```python
from build123d import *

# Parameters (mm, degrees)
F1_DEPTH = 30
F2_R     = 6.223398
F2_R_2   = 5.996206
F2_R_3   = 6.721343
F2_R_4   = 6.043049
F3_DEPTH = 35
F4_R     = 17.538538
F5_DEPTH = 500


with BuildPart() as f1:
    # F0 (on Front) → F1 (new body)
    with BuildSketch(Plane.XZ):
        with BuildLine():
            Line((-400.257468, -150.029927), (400.257468, -150.029927))
            ThreePointArc((400.257468, -150.029927), (550.287396, 0), (400.257468, 150.029927))
            Line((400.257468, 150.029927), (-400.257468, 150.029927))
            Line((-400.257468, 150.029927), (-400.257468, -150.029927))
        make_face()
    extrude(amount=F1_DEPTH)

    # F2 (on face) → F3 (cut)
    with BuildSketch(Plane.XZ.offset(30)):
        with Locations((-361.057468, 135.091782)):
            Circle(F2_R)
        with Locations((-361.057468, 104.35146)):
            Circle(F2_R_2)
        with Locations((-137.267468, 135.091782)):
            Circle(F2_R_3)
        with Locations((-137.267468, 104.35146)):
            Circle(F2_R_4)
    extrude(amount=-F3_DEPTH, mode=Mode.SUBTRACT)

    # F4 (on Top) → F5 (cut, symmetric)
    with BuildSketch(Plane.XY):
        with Locations((-400.190324, -14.999421)):
            Circle(F4_R)
    extrude(amount=F5_DEPTH, both=True, mode=Mode.SUBTRACT)


solid = f1.part
```
Design review of the part built by this model. Coordinates are the model's own, in mm. Coordinates: 2 decimals unless noted, no trailing zeros. Write each loop counter-clockwise with the first axis right and the second up, starting at its lowest first coordinate (ties: lowest second). Pieces come first, ordered by that corner, then holes. Notation, with made-up numbers: M 14,65 L 18,65 A29 cw 18,95 Z; hole C 71.25,39 d9. An arc over 180 degrees is marked long. Answer as a JSON object with one key per item and string values.
Item 1: Draft analysis for pull direction Y (two halves, no side actions). For faces 1 (the flat face through (-1, -15, -150.03)), 2 (the cylindrical face through (-382.654, -15.252, 2.1)), 3 (the flat face through (73, -30, 2)), state which applies: pulls with the +Y half, pulls with the -Y half, needs draft (parallel to the pull), parting line crosses it, or undercut.
Outcome:
{"face 1": "needs draft", "face 2": "undercut", "face 3": "pulls with the -Y half"}
Item 2: Insertion check: pin 1 Ø8 at (y, z) = (-9, -95.5) entering from -X; pin 2 Ø8 at (x, z) = (-137.27, 135.09) entering from -Y; pin 3 Ø8 at (y, z) = (-20, -6) entering from -X. Each pin has a flat end and moves straight along its axis. Give the tip position at first contact, or say it passes through.
Outcome:
{"pin 1": "x = -385.78", "pin 2": "through", "pin 3": "x = -385.14"}
Item 3: Add section B-B, the plane z = -90.5. Give the boundary of the cut face in (x, y), and give its area (3 significant figures).
Outcome:
{"outline": "M -391.1,-30 L 519.92,-30 L 519.92,0 L -391.1,0 A17.54 cw Z", "area": "27,200 mm²"}
Item 4: Add section A-A, the plane y = -19. Give the boundary of the cut face in (x, z).
Outcome:
{"outline": "M -383.11,-150.03 L 400.26,-150.03 A150.03 ccw 400.26,150.03 L -383.11,150.03 Z; hole C -361.06,135.09 d12.45; hole C -361.06,104.35 d11.99; hole C -137.27,135.09 d13.44; hole C -137.27,104.35 d12.09"}
Item 5: Add section C-C, the plane z = -131. Give the boundary of the cut face in (x, y), and give its area (3 significant figures).
Outcome:
{"outline": "M -391.1,-30 L 473.39,-30 L 473.39,0 L -391.1,0 A17.54 cw Z", "area": "25,800 mm²"}
Item 6: Wall thickness on probe 1 along X at (y, z) = (-14, 131); probe 2 along X at (y, z) = (-25.5, 138); probe 3 along X at (y, z) = (-1.5, 118.5): over which ranges is each line inside the solid? List them lowest first.
Outcome:
{"probe 1": "-382.68 to -365.75, -356.37 to -142.6, -131.94 to 473.39", "probe 2": "-386.14 to -366.56, -355.56 to -143.33, -131.21 to 459.12", "probe 3": "-388.99 to 492.27"}
